```python
from build123d import *

# Parameters (mm, degrees)
F0_R     = 31.75
F1_DEPTH = 6.35
F0_R_2   = 76.2
F0_R_3   = 74.4988936807
F2_DEPTH = 31.75


# Not quite as in the source:
# - a feature names something its author has since deleted; it is built from what else it names


with BuildPart() as f1:
    # F0 (on Front) → F1 (new body)
    with BuildSketch(Plane.XZ):
        with BuildLine():
            ThreePointArc((47.0428302523, -32.9697150499), (60.8100722022, -15.3863528649), (65.7145588579, 6.4002849501))
            ThreePointArc((65.7145588579, 6.4002849501), (65.7078231144, 7.227857987), (65.6876176686, 8.0552117454))
            Line((65.6876176686, 8.0552117454), (63.0200884494, 3.4349156071))
            ThreePointArc((63.0200884494, 3.4349156071), (60.4178100552, 2.7376372129), (59.720531661, 5.3399156071))
            Line((59.720531661, 5.3399156071), (65.0529232684, 14.5758887971))
            ThreePointArc((65.0529232684, 14.5758887971), (56.2331130755, 35.9675096944), (38.8466881833, 51.2352117455))
            Line((38.8466881833, 51.2352117455), (41.5142174026, 46.6149156071))
            ThreePointArc((41.5142174026, 46.6149156071), (40.8169390084, 44.0126372129), (38.2146606142, 44.7099156071))
            Line((38.2146606142, 44.7099156071), (32.8822690066, 53.9458887971))
            ThreePointArc((32.8822690066, 53.9458887971), (9.9466767851, 57.0035195621), (-11.9687534946, 49.5802849501))
            Line((-11.9687534946, 49.5802849501), (-6.6336950562, 49.5802849501))
            ThreePointArc((-6.6336950562, 49.5802849501), (-4.7286950562, 47.6752849501), (-6.6336950562, 45.7702849501))
            Line((-6.6336950562, 45.7702849501), (-17.2984782711, 45.7702849501))
            ThreePointArc((-17.2984782711, 45.7702849501), (-31.4142602999, 27.4362948179), (-35.9432656874, 4.7453581548))
            Line((-35.9432656874, 4.7453581548), (-33.2757364682, 9.3656542931))
            ThreePointArc((-33.2757364682, 9.3656542931), (-30.673458074, 10.0629326873), (-29.9761796798, 7.4606542931))
            Line((-29.9761796798, 7.4606542931), (-35.3085712873, -1.7753188969))
            ThreePointArc((-35.3085712873, -1.7753188969), (-26.4887610944, -23.1669397942), (-9.1023362022, -38.4346418453))
            Line((-9.1023362022, -38.4346418453), (-11.7698654214, -33.8143457069))
            ThreePointArc((-11.7698654214, -33.8143457069), (-11.0725870272, -31.2120673127), (-8.470308633, -31.9093457069))
            Line((-8.470308633, -31.9093457069), (-3.1379170255, -41.1453188969))
            ThreePointArc((-3.1379170255, -41.1453188969), (19.797675196, -44.202949662), (41.7131054758, -36.7797150499))
            Line((41.7131054758, -36.7797150499), (36.3780470374, -36.7797150499))
            ThreePointArc((36.3780470374, -36.7797150499), (34.4730470374, -34.8747150499), (36.3780470374, -32.9697150499))
            Line((36.3780470374, -32.9697150499), (47.0428302523, -32.9697150499))
        make_face()
        with Locations((14.8721759906, 6.4002849501)):
            Circle(F0_R, mode=Mode.SUBTRACT)
    extrude(amount=-F1_DEPTH)

    # F0 (on Front) → F2 (join)
    with BuildSketch(Plane.XZ):
        with Locations((14.8721759906, 6.4002849501)):
            Circle(F0_R_2)
        with Locations((14.8721759906, 6.4002849501)):
            Circle(F0_R_3, mode=Mode.SUBTRACT)
        with Locations((14.8721759906, 6.4002849501)):
            Circle(F0_R_3)
        with BuildLine():
            ThreePointArc((65.6876176686, 8.0552117454), (65.7078231144, 7.227857987), (65.7145588579, 6.4002849501))
            ThreePointArc((65.7145588579, 6.4002849501), (60.8100722022, -15.3863528649), (47.0428302523, -32.9697150499))
            Line((47.0428302523, -32.9697150499), (73.0397974374, -32.9697150499))
            ThreePointArc((73.0397974374, -32.9697150499), (74.9447974374, -34.8747150499), (73.0397974374, -36.7797150499))
            Line((73.0397974374, -36.7797150499), (41.7131054758, -36.7797150499))
            ThreePointArc((41.7131054758, -36.7797150499), (19.797675196, -44.202949662), (-3.1379170255, -41.1453188969))
            Line((-3.1379170255, -41.1453188969), (9.860566567, -63.6593529005))
            ThreePointArc((9.860566567, -63.6593529005), (9.1632881728, -66.2616312948), (6.5610097786, -65.5643529005))
            Line((6.5610097786, -65.5643529005), (-9.1023362022, -38.4346418453))
            ThreePointArc((-9.1023362022, -38.4346418453), (-26.4887610944, -23.1669397942), (-35.3085712873, -1.7753188969))
            Line((-35.3085712873, -1.7753188969), (-48.3070548798, -24.2893529005))
            ThreePointArc((-48.3070548798, -24.2893529005), (-50.909333274, -24.9866312948), (-51.6066116682, -22.3843529005))
            Line((-51.6066116682, -22.3843529005), (-35.9432656874, 4.7453581548))
            ThreePointArc((-35.9432656874, 4.7453581548), (-31.4142602999, 27.4362948179), (-17.2984782711, 45.7702849501))
            Line((-17.2984782711, 45.7702849501), (-43.2954454562, 45.7702849501))
            ThreePointArc((-43.2954454562, 45.7702849501), (-45.2004454562, 47.6752849501), (-43.2954454562, 49.5802849501))
            Line((-43.2954454562, 49.5802849501), (-11.9687534946, 49.5802849501))
            ThreePointArc((-11.9687534946, 49.5802849501), (9.9466767851, 57.0035195621), (32.8822690066, 53.9458887971))
            Line((32.8822690066, 53.9458887971), (19.8837854141, 76.4599228007))
            ThreePointArc((19.8837854141, 76.4599228007), (20.5810638083, 79.0622011949), (23.1833422025, 78.3649228007))
            Line((23.1833422025, 78.3649228007), (38.8466881833, 51.2352117455))
            ThreePointArc((38.8466881833, 51.2352117455), (56.2331130755, 35.9675096944), (65.0529232684, 14.5758887971))
            Line((65.0529232684, 14.5758887971), (78.051406861, 37.0899228007))
            ThreePointArc((78.051406861, 37.0899228007), (80.6536852552, 37.7872011949), (81.3509636494, 35.1849228007))
            Line((81.3509636494, 35.1849228007), (65.6876176686, 8.0552117454))
        make_face(mode=Mode.SUBTRACT)
    extrude(amount=-F2_DEPTH)


solid = f1.part
```
Input: part model. Units: mm. Frame: model coordinates. A direction names the side the tool comes from. Give positions to 0.01 mm unless a question says otherwise; leave off trailing zeros. Order: outer loops, then holes, each group sorted by start corner. A loop starts at its lowest first (then second) coordinate and runs counter-clockwise, first axis right, second up. Notation, with made-up numbers: (-12.75, 3.5) - (10.25, 3.5) arc R8 ccw to (10.25, 14.5) - close; hole circle Ø11 at (67, 7). An arc over 180 degrees is marked (long way). Put each result on its own line as item: value.
Item 1: Access query for faces 3 (the cylindrical face through (-4.73, 3.13, 47.72)), 4 (the cylindrical face through (56.042, 18.872, 36.233)). Directions: +Z, -Z, +X, -X, +Y, -Y. A direction counts if a zero-diameter tool reaches every point of the face in a straight line with its end or side. Return the directions, or none.
Found:
face 3: +Y, -Y
face 4: +Y
Item 2: Section query B-B, the plane x = 13. Return loops of the section in (y, z), then the cut area to 3 significant figures.
Found:
outline: (0, -69.78) - (31.75, -69.78) - (31.75, -44.41) - (6.35, -44.41) - (6.35, -25.29) - (0, -25.29) - close; (0, 38.1) - (6.35, 38.1) - (6.35, 57.21) - (31.75, 57.21) - (31.75, 82.58) - (0, 82.58) - close
area: 1,850 mm^2
Item 3: Section query C-C, the plane y = 23. Return loops of the section in (x, z) (3 decimals).
Found:
outline: circle Ø152.4 at (14.872, 6.4); hole (-51.607, -22.384) arc R1.905 ccw to (-48.307, -24.289) - (-35.309, -1.775) arc R50.842 ccw to (-9.102, -38.435) - (6.561, -65.564) arc R1.905 ccw to (9.861, -63.659) - (-3.138, -41.145) arc R50.842 ccw to (41.713, -36.78) - (73.04, -36.78) arc R1.905 ccw to (73.04, -32.97) - (47.043, -32.97) arc R50.842 ccw to (65.688, 8.055) - (81.351, 35.185) arc R1.905 ccw to (78.051, 37.09) - (65.053, 14.576) arc R50.842 ccw to (38.847, 51.235) - (23.183, 78.365) arc R1.905 ccw to (19.884, 76.46) - (32.882, 53.946) arc R50.842 ccw to (-11.969, 49.58) - (-43.295, 49.58) arc R1.905 ccw to (-43.295, 45.77) - (-17.298, 45.77) arc R50.842 ccw to (-35.943, 4.745) - close
Item 4: Ray query, L1, parallel to X at y = 21.5, z = 37; L2, parallel to X at y = 27, z = 27.5; L3, parallel to Z at x = 65.5, y = 5. Return the intervals inside material, ascending. Write a range as from..to.
Found:
L1: x = -54.91..-25.73, 55.48..78, 81.4..84.66
L2: x = -58.35..-31.39, 61.13..72.51, 76.91..88.09
L3: z = -50.55..-36.78, -32.97..7.73, 15.35..63.35
Item 5: Contact query for flat-ended pins moving along their axis: pin 1 (12 mm diameter, centred on x = 26, y = 26, fed in from -Z); pin 2 (4 mm diameter, centred on y = 4.5, z = -11.5, fed in from -X); pin 3 (4 mm diameter, centred on y = 12.5, z = 33.5, fed in from -X). Output: stop coordinate, or through.
Found:
pin 1: stops at z = -69.63
pin 2: stops at x = -59.65
pin 3: stops at x = -57.08
Item 6: Section query D-D, the plane z = 69. Return loops of the section in (x, y), then the cut area to 3 significant figures.
Found:
outline: (-28.58, 0) - (24.19, 0) - (24.19, 31.75) - (-28.58, 31.75) - close; (28.59, 0) - (58.32, 0) - (58.32, 31.75) - (28.59, 31.75) - close
area: 2,620 mm^2
Item 7: Section query A-A, the plane y = 4. Return loops of the section in (x, z) (3 decimals), then the cut area to 3 significant figures.
Found:
outline: circle Ø152.4 at (14.872, 6.4); hole (-51.607, -22.384) arc R1.905 ccw to (-48.307, -24.289) - (-29.976, 7.461) arc R1.905 ccw to (-33.276, 9.366) - close; hole (-43.295, 45.77) - (-6.634, 45.77) arc R1.905 ccw to (-6.634, 49.58) - (-43.295, 49.58) arc R1.905 ccw to start; hole circle Ø63.5 at (14.872, 6.4); hole (-11.77, -33.814) - (6.561, -65.564) arc R1.905 ccw to (9.861, -63.659) - (-8.47, -31.909) arc R1.905 ccw to start; hole (19.884, 76.46) - (38.215, 44.71) arc R1.905 ccw to (41.514, 46.615) - (23.183, 78.365) arc R1.905 ccw to start; hole (36.378, -36.78) - (73.04, -36.78) arc R1.905 ccw to (73.04, -32.97) - (36.378, -32.97) arc R1.905 ccw to start; hole (59.721, 5.34) arc R1.905 ccw to (63.02, 3.435) - (81.351, 35.185) arc R1.905 ccw to (78.051, 37.09) - close
area: 14,200 mm^2
Item 8: Draft query along X for faces 1 (the cylindrical face through (60.45, 3.13, 2.72)), 2 (the cylindrical face through (-1.6, 15.7, -68)). Return one class per face: +X half, -X half, draft (parallel to the pull), parting line (faces both ways), or undercut.
Found:
face 1: undercut
face 2: parting line
